```python
from build123d import *

# Parameters (mm, degrees)
EXTRUDE_1_DEPTH     = 15
SKETCH_2_R          = 1.5
CUT_EXTRUDE_1_DEPTH = 44.847690931
SKETCH_3_R          = 7.75
CUT_EXTRUDE_2_DEPTH = 5
SKETCH_4_W          = 15.5
SKETCH_4_H          = 5.5
SKETCH_5_W          = 88.652710044
SKETCH_5_H          = 26.513310491
CUT_EXTRUDE_3_DEPTH = 44.847690931
SKETCH_6_R          = 2.5
CUT_EXTRUDE_4_DEPTH = 44.847690931
FILLET_3_R          = 1
FILLET_4_R          = 1
FILLET_5_R          = 3


with BuildPart() as part:
    # 草圖1 → 填料-伸長1 (new body)
    with BuildSketch(Plane.XY):
        with BuildLine():
            Line((-29.9, 21.9), (29.9, 21.9))
            ThreePointArc((29.9, 21.9), (33.435533906, 20.435533906), (34.9, 16.9))
            Line((34.9, 16.9), (34.9, -16.9))
            ThreePointArc((34.9, -16.9), (33.435533906, -20.435533906), (29.9, -21.9))
            Line((29.9, -21.9), (-29.9, -21.9))
            ThreePointArc((-29.9, -21.9), (-33.435533906, -20.435533906), (-34.9, -16.9))
            Line((-34.9, -16.9), (-34.9, 16.9))
            ThreePointArc((-34.9, 16.9), (-33.435533906, 20.435533906), (-29.9, 21.9))
        make_face()
    extrude(amount=EXTRUDE_1_DEPTH)

    # 草圖2 → 除料-伸長1 (cut, through all)
    with BuildSketch(Plane.XY.offset(15)):
        with Locations((-32.4, 11.9)):
            Circle(SKETCH_2_R)
        with Locations(Location((-32.4, -11.9, 0), (0, 0, 180))):
            Circle(SKETCH_2_R)
        with Locations((32.4, -11.9)):
            Circle(SKETCH_2_R)
        with Locations(Location((32.4, 11.9, 0), (0, 0, 180))):
            Circle(SKETCH_2_R)
    extrude(amount=-CUT_EXTRUDE_1_DEPTH, mode=Mode.SUBTRACT)

    # 草圖3 → 除料-伸長2 (cut)
    with BuildSketch(Plane.XY.offset(15)):
        Circle(SKETCH_3_R)
    extrude(amount=-CUT_EXTRUDE_2_DEPTH, mode=Mode.SUBTRACT)

    # 草圖4 → 除料-旋轉1 (revolve, cut)
    with BuildSketch(Plane(origin=(0, 0, 0), x_dir=(1, 0, 0), z_dir=(0, 1, 0)), mode=Mode.PRIVATE) as cut_revolve_1_sk:
        with Locations((-7.75, -7.25)):
            Rectangle(SKETCH_4_W, SKETCH_4_H)
    revolve(cut_revolve_1_sk.sketch.rotate(Axis((0, 0, 15), (0, 0, -1)), 180), axis=Axis((0, 0, 15), (0, 0, -1)), mode=Mode.SUBTRACT)

    # 草圖5 → 除料-伸長3 (cut, through all)
    with BuildSketch(Plane.XY.offset(15)):
        with Locations((0.900027513, -13.256655246)):
            Rectangle(SKETCH_5_W, SKETCH_5_H)
    extrude(amount=-CUT_EXTRUDE_3_DEPTH, mode=Mode.SUBTRACT)

    # 草圖6 → 除料-伸長4 (cut, through all)
    with BuildSketch(Plane(origin=(0, 21.9, 0), x_dir=(1, 0, 0), z_dir=(0, 1, 0))):
        with Locations(Location((-22.9, -7.5, 0), (0, 0, 270))):
            Circle(SKETCH_6_R)
        with Locations(Location((22.9, -7.5, 0), (0, 0, 90))):
            Circle(SKETCH_6_R)
    extrude(amount=-CUT_EXTRUDE_4_DEPTH, mode=Mode.SUBTRACT)

    # 圓角3
    fillet_3_edges = [part.edges().sort_by_distance(p)[0] for p in [
        (0, 15.5, 10),
        (0, 15.5, 4.5),
    ]]
    fillet(fillet_3_edges, radius=FILLET_3_R)

    # 圓角4
    fillet_4_edges = [part.edges().sort_by_distance(p)[0] for p in [
        (0, 7.75, 15),
    ]]
    fillet(fillet_4_edges, radius=FILLET_4_R)

    # 圓角5
    fillet_5_edges = [part.edges().sort_by_distance(p)[0] for p in [
        (0, 7.75, 10),
    ]]
    fillet(fillet_5_edges, radius=FILLET_5_R)


solid = part.part
```
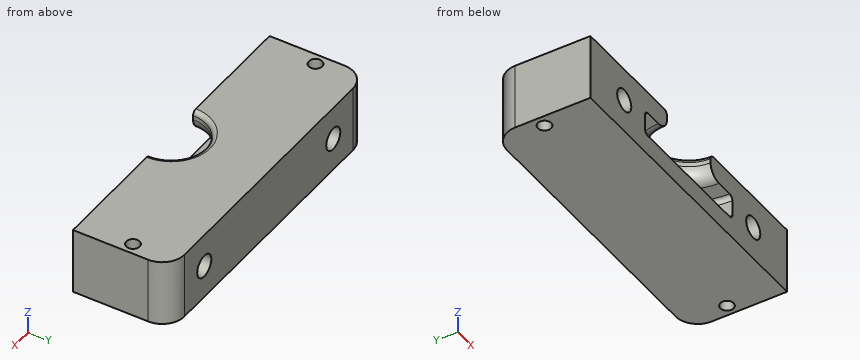
Here's how the part is built. I have some questions about the finished solid (model axes, mm). Coordinates: 2 decimals unless noted, no trailing zeros. Write each loop counter-clockwise with the first axis right and the second up, starting at its lowest first coordinate (ties: lowest second). Pieces come first, ordered by that corner, then holes. Notation, with made-up numbers: M 14.25,51.25 L 65.25,51.25 A13 ccw 65.25,74.25 Z; hole C -34.5,24 d10. An arc over 180 degrees is marked long. Answer as CSV lines item,"result". Start each with the question number.
Q1. Suppose I cut it at C-C, the plane z = 8. List the corners of the cut face in (x, y) for me.
Q2. Suppose I cut it at D-D, the plane y = 11.9. State how many separate pieces and enclosed holes the cut face has, then the cut area to 3 significant figures.
Q3. Suppose I cut it at A-A, the plane x = 22.9. List the corners of the cut face in (y, z) for me, then the cut area to 3 significant figures.
Q4. Suppose I cut it at B-B, the plane z = 3.5. List the corners of the cut face in (x, y) for me, then the cut area to 3 significant figures.
Q5. I need wall thicknesses on probe 1 along Z at (x, y) = (22.9, 12.5); probe 2 along Z at (x, y) = (10.5, 3.25); probe 3 along Z at (x, y) = (-4.5, 1.25). Which ranges of each line are inside material? Lowest first, please. Write a range as [from, to].
Q6. Will this pin go through, and if not, where does the flat tip stop? pin 1 Ø4.5 at (x, y) = (0.5, 4) entering from +Z.
Entries:
1,outline,"M -34.9,0 L -25.35,0 L -25.35,21.9 L -29.9,21.9 A5 ccw -34.9,16.9 Z; M -20.45,0 L -15.5,0 A15.5 cw 15.5,0 L 20.45,0 L 20.45,21.9 L -20.45,21.9 Z; M 25.35,0 L 34.9,0 L 34.9,16.9 A5 ccw 29.9,21.9 L 25.35,21.9 Z; hole C -32.4,11.9 d3; hole C 32.4,11.9 d3"
2,separate pieces,"3"
2,enclosed holes,"3"
2,area,"810 mm²"
3,outline,"M 0,0 L 21.9,0 L 21.9,5 L 0,5 Z; M 0,10 L 21.9,10 L 21.9,15 L 0,15 Z"
3,area,"219 mm²"
4,outline,"M -34.9,0 L 34.9,0 L 34.9,16.9 A5 ccw 29.9,21.9 L -29.9,21.9 A5 ccw -34.9,16.9 Z; hole C -32.4,11.9 d3; hole C 32.4,11.9 d3"
4,area,"1,500 mm²"
5,probe 1,"z = [0, 5], [10, 15]"
5,probe 2,"z = [0, 4.5], [10, 15]"
5,probe 3,"z = [0, 4.5]"
6,pin 1,"stops at z = 4.5"
